Could you check a few things on this model? Use its own coordinates, in mm. Give positions to 0.01 mm unless a question says otherwise; leave off trailing zeros. Order: outer loops, then holes, each group sorted by start corner. A loop starts at its lowest first (then second) coordinate and runs counter-clockwise, first axis right, second up. Notation, with made-up numbers: (67, -9.75) - (86, -9.75) arc R16 ccw to (86, 10.25) - close; hole circle Ø9 at (22.5, -31.75). An arc over 180 degrees is marked (long way). Put each result on its own line as item: value.
from build123d import *

# Parameters (mm, degrees)
SKETCH_1_R      = 1.7
SKETCH_1_W      = 3
SKETCH_1_H      = 5
SKETCH_1_W_2    = 5
SKETCH_1_H_2    = 3
EXTRUDE_1_DEPTH = 3


with BuildPart() as part:
    # 草图1 → 凸台-拉伸1 (new body)
    with BuildSketch(Plane(origin=(0, 0, 0), x_dir=(1, 0, 0), z_dir=(0, 1, 0))):
        with BuildLine():
            Line((54, 24), (70, 24))
            ThreePointArc((70, 24), (0, 74), (-70, 24))
            Line((-70, 24), (-54, 24))
            Line((-54, 24), (-54, -24))
            Line((-54, -24), (-70, -24))
            ThreePointArc((-70, -24), (0, -74), (70, -24))
            Line((70, -24), (54, -24))
            Line((54, -24), (54, 24))
        make_face()
        with Locations(Location((-49.497474683, -49.497474683, 0), (0, 0, 270))):
            Circle(SKETCH_1_R, mode=Mode.SUBTRACT)
        with Locations(Location((-5, -68, 0), (0, 0, 270))):
            Circle(SKETCH_1_R, mode=Mode.SUBTRACT)
        with Locations(Location((-42, -8, 0), (0, 0, 270))):
            Circle(SKETCH_1_R, mode=Mode.SUBTRACT)
        with Locations((-34, -35.5)):
            Rectangle(SKETCH_1_W, SKETCH_1_H, mode=Mode.SUBTRACT)
        with Locations(Location((-28, -8, 0), (0, 0, 270))):
            Circle(SKETCH_1_R, mode=Mode.SUBTRACT)
        with Locations(Location((5, -68, 0), (0, 0, 270))):
            Circle(SKETCH_1_R, mode=Mode.SUBTRACT)
        with Locations((0, -63.5)):
            Rectangle(SKETCH_1_W_2, SKETCH_1_H_2, mode=Mode.SUBTRACT)
        with Locations(Location((49.497474683, -49.497474683, 0), (0, 0, 270))):
            Circle(SKETCH_1_R, mode=Mode.SUBTRACT)
        with Locations((34, -35.5)):
            Rectangle(SKETCH_1_W, SKETCH_1_H, mode=Mode.SUBTRACT)
        with Locations(Location((28, -8, 0), (0, 0, 270))):
            Circle(SKETCH_1_R, mode=Mode.SUBTRACT)
        with Locations(Location((42, -8, 0), (0, 0, 270))):
            Circle(SKETCH_1_R, mode=Mode.SUBTRACT)
        with Locations(Location((-42, 8, 0), (0, 0, 270))):
            Circle(SKETCH_1_R, mode=Mode.SUBTRACT)
        with Locations(Location((-28, 8, 0), (0, 0, 270))):
            Circle(SKETCH_1_R, mode=Mode.SUBTRACT)
        with Locations(Location((-34.15, 30, 0), (0, 0, 270))):
            Circle(SKETCH_1_R, mode=Mode.SUBTRACT)
        with Locations(Location((0, 30, 0), (0, 0, 270))):
            Circle(SKETCH_1_R, mode=Mode.SUBTRACT)
        with Locations(Location((-49.497474683, 49.497474683, 0), (0, 0, 270))):
            Circle(SKETCH_1_R, mode=Mode.SUBTRACT)
        with Locations(Location((-5, 68, 0), (0, 0, 270))):
            Circle(SKETCH_1_R, mode=Mode.SUBTRACT)
        with BuildLine():
            Line((4.5, -7.5), (-4.5, -7.5))
            ThreePointArc((-4.5, -7.5), (-6.621320344, -6.621320344), (-7.5, -4.5))
            Line((-7.5, -4.5), (-7.5, 4.5))
            ThreePointArc((-7.5, 4.5), (-6.621320344, 6.621320344), (-4.5, 7.5))
            Line((-4.5, 7.5), (4.5, 7.5))
            ThreePointArc((4.5, 7.5), (6.621320344, 6.621320344), (7.5, 4.5))
            Line((7.5, 4.5), (7.5, -4.5))
            ThreePointArc((7.5, -4.5), (6.621320344, -6.621320344), (4.5, -7.5))
        make_face(mode=Mode.SUBTRACT)
        with Locations(Location((28, 8, 0), (0, 0, 270))):
            Circle(SKETCH_1_R, mode=Mode.SUBTRACT)
        with Locations(Location((34.15, 30, 0), (0, 0, 270))):
            Circle(SKETCH_1_R, mode=Mode.SUBTRACT)
        with Locations(Location((42, 8, 0), (0, 0, 270))):
            Circle(SKETCH_1_R, mode=Mode.SUBTRACT)
        with Locations(Location((5, 68, 0), (0, 0, 270))):
            Circle(SKETCH_1_R, mode=Mode.SUBTRACT)
        with Locations(Location((49.497474683, 49.497474683, 0), (0, 0, 270))):
            Circle(SKETCH_1_R, mode=Mode.SUBTRACT)
    extrude(amount=EXTRUDE_1_DEPTH)


solid = part.part
1) Suppose I cut it at B-B, the plane x = 42. List the corners of the cut face in (y, z) for me, and give its area (3 significant figures).
Filled in:
outline: (0, -60.93) - (3, -60.93) - (3, -9.7) - (0, -9.7) - close; (0, -6.3) - (3, -6.3) - (3, 6.3) - (0, 6.3) - close; (0, 9.7) - (3, 9.7) - (3, 60.93) - (0, 60.93) - close
area: 345 mm^2
2) We'd pull the mould along Z, two halves only. Please class faces 1 (the cylindrical face through (5.07, 1.48, 66.3)), 2 (the cylindrical face through (1.29, 1.48, -73.99)), 3 (the cylindrical face through (-1.29, 1.48, 73.99)), 4 (the cylindrical face through (-26.314, 1.479, -8.221)): pulls with the +Z half, pulls with the -Z half, needs draft (parallel to the pull), parting line crosses it, or undercut.
Filled in:
face 1: undercut
face 2: pulls with the -Z half
face 3: pulls with the +Z half
face 4: undercut
3) Suppose I cut it at D-D, the plane y = 0.7. State how many separate pieces and enclosed holes the cut face has, and give its area (3 significant figures).
Filled in:
separate pieces: 1
enclosed holes: 23
area: 15,000 mm^2
4) Suppose I cut it at A-A, the plane x = 0. List the corners of the cut face in (y, z) for me.
Filled in:
outline: (0, -74) - (3, -74) - (3, -31.7) - (0, -31.7) - close; (0, -28.3) - (3, -28.3) - (3, -7.5) - (0, -7.5) - close; (0, 7.5) - (3, 7.5) - (3, 62) - (0, 62) - close; (0, 65) - (3, 65) - (3, 74) - (0, 74) - close
5) If I drill on line 1 (X direction, y = 1.35, z = 8); line 2 (X direction, y = 0.9, z = 15); line 3 (Z direction, x = 1, y = 2.2), over which ranges is the centre line in solid material (lowest first)? Write a range as [from, to].
Filled in:
line 1: x = [-54, -43.7], [-40.3, -29.7], [-26.3, 26.3], [29.7, 40.3], [43.7, 54]
line 2: x = [-54, 54]
line 3: z = [-73.99, -31.37], [-28.63, -7.5], [7.5, 62], [65, 73.99]
6) Suppose I cut it at C-C, the plane z = -68. List the corners of the cut face in (x, y) for me.
Filled in:
outline: (-29.19, 0) - (-6.7, 0) - (-6.7, 3) - (-29.19, 3) - close; (-3.3, 0) - (3.3, 0) - (3.3, 3) - (-3.3, 3) - close; (6.7, 0) - (29.19, 0) - (29.19, 3) - (6.7, 3) - close
7) I'm going to push flat-ended pins straight in: pin 1 (1 mm diameter, centred on y = 1, z = 2, fed in from +X); pin 2 (1 mm diameter, centred on y = 1, z = 36.5, fed in from +X); pin 3 (1.5 mm diameter, centred on x = 26.5, y = 1, fed in from -Z). Where does each tip first touch, or does it pass through?
Filled in:
pin 1: stops at x = 54
pin 2: stops at x = 64.65
pin 3: stops at z = -69.38
